Read the model definition and answer for the solid it produces. Units are mm, in the model's axes. Round coordinates to 2 decimals unless told otherwise and drop trailing zeros. Loops run counter-clockwise (first coordinate to the right, second up) from the corner with the lowest first, then second, coordinate; pieces in that order, holes last. Notation, with made-up numbers: (67, 49) - (126, 49) arc R4 ccw to (126, 54) - close; hole circle Ø6 at (59.25, 65). An arc over 180 degrees is marked (long way). Use CSV: the item, a comma, the result in double quotes. Start each with the question number.
1. Determine the mould class of faces 1 (the cylindrical face through (1.012, -17.196, 1.972)), 2 (the flat face through (38, 23, 4)), 3 (the flat face through (38, 69.5, 2)) for opening direction Y: +Y half, -Y half, draft (parallel to the pull), parting line (faces both ways), or undercut.
2. Find section D-D (y = 32.5). Give the vertices of the cut face in (x, z), and give its area (3 significant figures).
3. Find section B-B (x = 59). Give the vertices of the cut face in (y, z), and give its area (3 significant figures).
4. Consider line 1 along Y through (x, z) = (76.5, 0.9); line 2 along Y through (x, z) = (16.5, 0.5); line 3 along Z through (x, y) = (62, 33). Determine where each line is inside the solid, lowest interval first.
5. Given pin 1 Ø4.5 at (x, y) = (19, 32.5) entering from +Z; pin 2 Ø2 at (x, y) = (59, 32.5) entering from +Z; pin 3 Ø4.5 at (x, y) = (59, 12.5) entering from -Z, each flat-ended and moving along its own axis, determine where each tip first touches the part or whether it passes through.
6. Find section A-A (y = -15). Give the vertices of the cut face in (x, z).
7. Find section C-C (x = 76.5). Give the vertices of the cut face in (y, z), and give its area (3 significant figures).
from build123d import *

# Parameters (mm, degrees)
SKETCH1_W           = 78
SKETCH1_H           = 45
SKETCH1_R           = 1.6
BOSS_EXTRUDE1_DEPTH = 4
SKETCH5_W           = 94
SKETCH5_H           = 94
SKETCH5_R           = 2.25
BOSS_EXTRUDE3_DEPTH = 4
SKETCH6_R           = 1.65
CUT_EXTRUDE1_DEPTH  = 5
CHAMFER1_SIZE       = 1.6


with BuildPart() as part:
    # Sketch1 → Boss-Extrude1 (new body)
    with BuildSketch(Plane.XY):
        with Locations((39, 22.5)):
            Rectangle(SKETCH1_W, SKETCH1_H)
        with Locations((19, 32.5)):
            Circle(SKETCH1_R, mode=Mode.SUBTRACT)
        with Locations((59, 32.5)):
            Circle(SKETCH1_R, mode=Mode.SUBTRACT)
        with Locations((59, 12.5)):
            Circle(SKETCH1_R, mode=Mode.SUBTRACT)
        with Locations((19, 12.5)):
            Circle(SKETCH1_R, mode=Mode.SUBTRACT)
    extrude(amount=BOSS_EXTRUDE1_DEPTH)

    # Sketch5 → Boss-Extrude3 (add)
    with BuildSketch(Plane.XY):
        with Locations((39, 22.5)):
            Rectangle(SKETCH5_W, SKETCH5_H)
        with Locations((1.5, 60)):
            Circle(SKETCH5_R, mode=Mode.SUBTRACT)
        with Locations((76.5, 60)):
            Circle(SKETCH5_R, mode=Mode.SUBTRACT)
        with Locations((76.5, -15)):
            Circle(SKETCH5_R, mode=Mode.SUBTRACT)
        with Locations((1.5, -15)):
            Circle(SKETCH5_R, mode=Mode.SUBTRACT)
    extrude(amount=BOSS_EXTRUDE3_DEPTH)

    # Sketch6 → Cut-Extrude1 (cut, through all)
    with BuildSketch(Plane(origin=(0, 0, 0), x_dir=(-1, 0, 0), z_dir=(0, 0, -1))):
        with Locations((-59, 32.5)):
            Circle(SKETCH6_R)
        with Locations((-59, 12.5)):
            Circle(SKETCH6_R)
        with Locations((-19, 12.5)):
            Circle(SKETCH6_R)
        with Locations((-19, 32.5)):
            Circle(SKETCH6_R)
    extrude(amount=-CUT_EXTRUDE1_DEPTH, mode=Mode.SUBTRACT)

    # Chamfer1
    chamfer1_edges = [part.edges().sort_by_distance(p)[0] for p in [
        (20.65, 32.5, 0),
        (20.65, 12.5, 0),
        (60.65, 12.5, 0),
        (60.65, 32.5, 0),
    ]]
    chamfer(chamfer1_edges, length=CHAMFER1_SIZE)


solid = part.part
Filled sheet:
1,face 1,"undercut"
1,face 2,"draft"
1,face 3,"+Y half"
2,outline,"(-8, 0) - (15.75, 0) - (17.35, 1.6) - (17.35, 4) - (-8, 4) - close; (20.65, 1.6) - (22.25, 0) - (55.75, 0) - (57.35, 1.6) - (57.35, 4) - (20.65, 4) - close; (60.65, 1.6) - (62.25, 0) - (86, 0) - (86, 4) - (60.65, 4) - close"
2,area,"344 mm²"
3,outline,"(-24.5, 0) - (9.25, 0) - (10.85, 1.6) - (10.85, 4) - (-24.5, 4) - close; (14.15, 1.6) - (15.75, 0) - (29.25, 0) - (30.85, 1.6) - (30.85, 4) - (14.15, 4) - close; (34.15, 1.6) - (35.75, 0) - (69.5, 0) - (69.5, 4) - (34.15, 4) - close"
3,area,"344 mm²"
4,line 1,"y = -24.5 to -17.25, -12.75 to 57.75, 62.25 to 69.5"
4,line 2,"y = -24.5 to 11.35, 13.65 to 31.35, 33.65 to 69.5"
4,line 3,"z = 0.21 to 4"
5,pin 1,"stops at z = 4"
5,pin 2,"passes through"
5,pin 3,"stops at z = 1"
6,outline,"(-8, 0) - (-0.75, 0) - (-0.75, 4) - (-8, 4) - close; (3.75, 0) - (74.25, 0) - (74.25, 4) - (3.75, 4) - close; (78.75, 0) - (86, 0) - (86, 4) - (78.75, 4) - close"
7,outline,"(-24.5, 0) - (-17.25, 0) - (-17.25, 4) - (-24.5, 4) - close; (-12.75, 0) - (57.75, 0) - (57.75, 4) - (-12.75, 4) - close; (62.25, 0) - (69.5, 0) - (69.5, 4) - (62.25, 4) - close"
7,area,"340 mm²"
